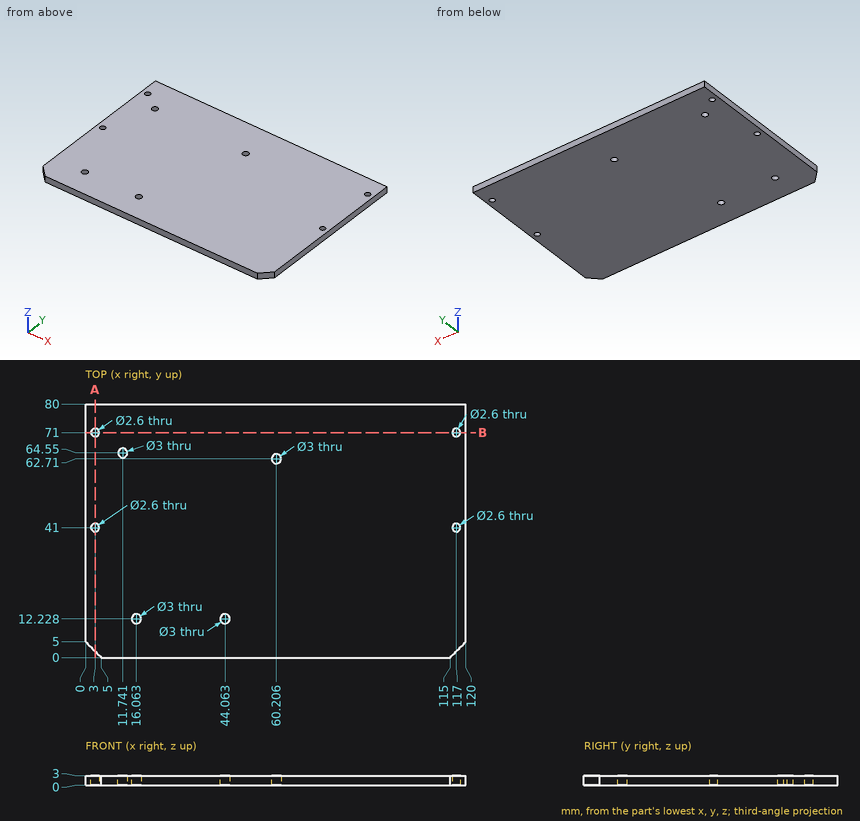
Source: three-view drawing plus pictorial views. Frame: mm from the lowest corner of the part. Round coordinates to 2 decimals unless told otherwise and drop trailing zeros. Order: outer loops, then holes, each group sorted by start corner. A loop starts at its lowest first (then second) coordinate and runs counter-clockwise, first axis right, second up. Notation, with made-up numbers: (85, 44) -> (115, 44) arc R9 cw to (115, 52) -> close; hole circle Ø5 at (-12, 13.5). An arc over 180 degrees is marked (long way). Use one line per item in the form item = value. Start each with the question number.
1. Line query: probe 1 along X at (y, z) = (71, 1.4); probe 2 along Y at (x, z) = (117, 1.8); probe 3 along X at (y, z) = (41.5, 1.9). Output: solid intervals per line, ascending.
2. Cut plane A-A (x = 3). Return the cut outline in (y, z).
3. Cut plane B-B (y = 71). Return the cut outline in (x, z).
Solution:
q1.probe_1 = 0 to 1.7, 4.3 to 115.7, 118.3 to 120
q1.probe_2 = 2 to 39.7, 42.3 to 69.7, 72.3 to 80
q1.probe_3 = 0 to 1.8, 4.2 to 115.8, 118.2 to 120
q2.outline = (2, 0) -> (39.7, 0) -> (39.7, 3) -> (2, 3) -> close; (42.3, 0) -> (69.7, 0) -> (69.7, 3) -> (42.3, 3) -> close; (72.3, 0) -> (80, 0) -> (80, 3) -> (72.3, 3) -> close
q3.outline = (0, 0) -> (1.7, 0) -> (1.7, 3) -> (0, 3) -> close; (4.3, 0) -> (115.7, 0) -> (115.7, 3) -> (4.3, 3) -> close; (118.3, 0) -> (120, 0) -> (120, 3) -> (118.3, 3) -> close
